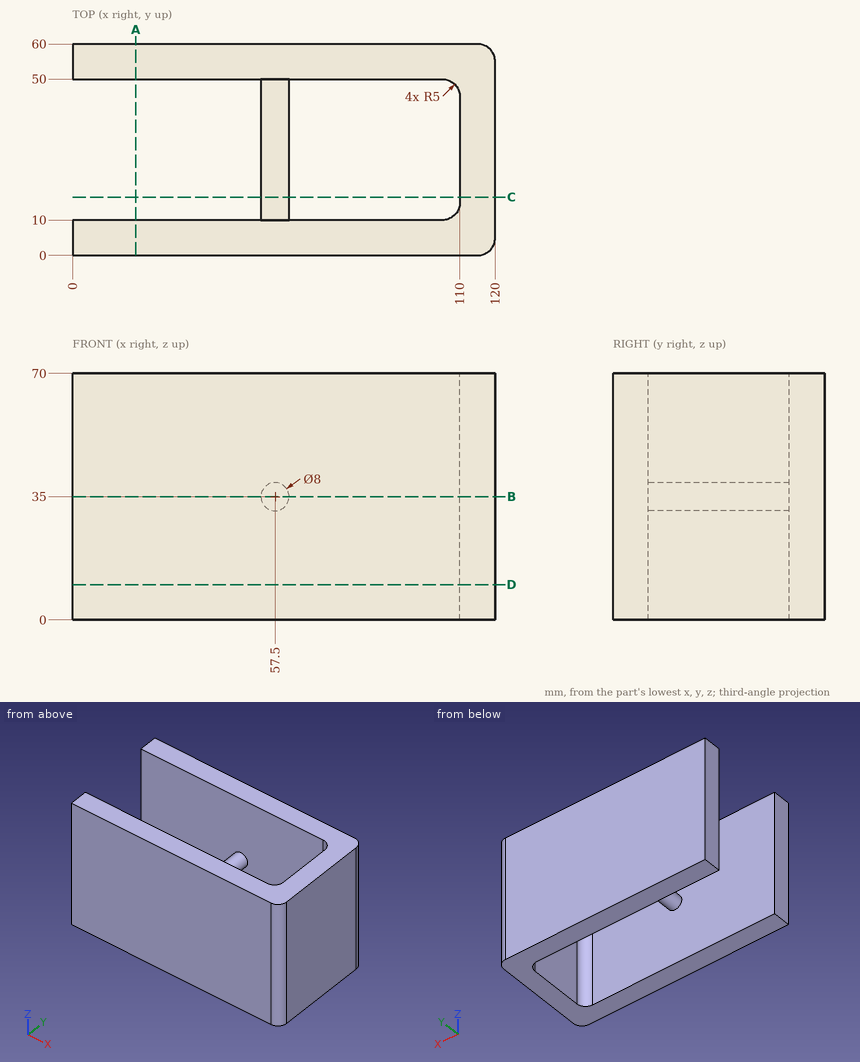
Check sheet for the drawn part. Datum: minimum x, y, z corner. Units: mm. Round coordinates to 2 decimals unless told otherwise and drop trailing zeros. Order: outer loops, then holes, each group sorted by start corner. A loop starts at its lowest first (then second) coordinate and runs counter-clockwise, first axis right, second up. Notation, with made-up numbers: M -35.75,62.5 L -11.75,62.5 A22 ccw -11.75,81.5 Z; hole C 56.25,88.25 d6. An arc over 180 degrees is marked long. Write each question's results on one line, items separated by ' | '. Start each with the question number.
1. Go/stop test with flat-tipped pins: P1, Ø1.5, axis at y = 18.5, z = 38.5, coming from the -X side; P2, Ø15, axis at y = 29.5, z = 46, coming from the -X side. Record where each tip stops, or that it passes through.
2. Cross-section at D-D on z = 10. Record the boundary of the cut face in (x, y), plus the area to 3 significant figures.
3. Material ranges on L1, parallel to Y at x = 83.5, z = 44; L2, parallel to X at y = 45, z = 25; L3, parallel to X at y = 14, z = 24, recorded low to high. Write a range as from..to.
4. Cross-section at C-C on y = 16.5. Record the boundary of the cut face in (x, z).
5. Cross-section at B-B on z = 35. Record the boundary of the cut face in (x, y).
6. Cross-section at A-A on x = 18. Record the boundary of the cut face in (y, z).
Resolved:
1) P1: x = 54.6 | P2: x = 55.56
2) outline: M 0,0 L 115,0 A5 ccw 120,5 L 120,55 A5 ccw 115,60 L 0,60 L 0,50 L 105,50 A5 cw 110,45 L 110,15 A5 cw 105,10 L 0,10 Z | area: 2,800 mm2
3) L1: 0..10, 50..60 | L2: 110..120 | L3: 109.9..120
4) outline: C 57.5,35 d8; M 110,0 L 120,0 L 120,70 L 110,70 Z
5) outline: M 0,0 L 115,0 A5 ccw 120,5 L 120,55 A5 ccw 115,60 L 0,60 L 0,50 L 53.5,50 L 53.5,10 L 0,10 Z; hole M 61.5,10 L 105,10 A5 ccw 110,15 L 110,45 A5 ccw 105,50 L 61.5,50 Z
6) outline: M 0,0 L 10,0 L 10,70 L 0,70 Z; M 50,0 L 60,0 L 60,70 L 50,70 Z
